```python
from build123d import *

# Parameters (mm, degrees)
EXTRUDE_1_DEPTH     = 3
SKETCH_2_R          = 1.6
CUT_EXTRUDE_1_DEPTH = 26.184320519
SKETCH_4_W          = 14
SKETCH_4_H          = 8
EXTRUDE_2_DEPTH     = 14.55
SKETCH_5_W          = 8
SKETCH_5_H          = 14.55
CUT_EXTRUDE_2_DEPTH = 32.452384647
SKETCH_6_R          = 1.05
CUT_EXTRUDE_3_DEPTH = 37.404017635
FILLET_1_R          = 3
RIB_1_REACH         = 32.549
SKETCH_7_WALL_W     = 71.642367062
SKETCH_7_WALL_H     = 3
RIB_2_REACH         = 32.549
SKETCH_8_WALL_W     = 71.642367062
SKETCH_8_WALL_H     = 3


with BuildPart() as part:
    # 草图1 → 凸台-拉伸1 (new body)
    with BuildSketch(Plane.XY):
        with BuildLine():
            Line((-21.779069767, 2.986991809), (-0.465116279, 4.978319681))
            ThreePointArc((-0.465116279, 4.978319681), (0, 5), (0.465116279, 4.978319681))
            Line((0.465116279, 4.978319681), (21.779069767, 2.986991809))
            ThreePointArc((21.779069767, 2.986991809), (24.5, 0), (21.779069767, -2.986991809))
            Line((21.779069767, -2.986991809), (0.465116279, -4.978319681))
            ThreePointArc((0.465116279, -4.978319681), (0, -5), (-0.465116279, -4.978319681))
            Line((-0.465116279, -4.978319681), (-21.779069767, -2.986991809))
            ThreePointArc((-21.779069767, -2.986991809), (-24.5, 0), (-21.779069767, 2.986991809))
        make_face()
    extrude(amount=EXTRUDE_1_DEPTH)

    # 草图2 → 切除-拉伸1 (cut, through all)
    with BuildSketch(Plane.XY.offset(3)):
        with Locations((-20, 0)):
            Circle(SKETCH_2_R)
        with Locations((20, 0)):
            Circle(SKETCH_2_R)
    extrude(amount=-CUT_EXTRUDE_1_DEPTH, mode=Mode.SUBTRACT)

    # 草图4 → 凸台-拉伸2 (add)
    with BuildSketch(Plane.XY.offset(3)):
        Rectangle(SKETCH_4_W, SKETCH_4_H)
    extrude(amount=EXTRUDE_2_DEPTH)

    # 草图5 → 切除-拉伸2 (cut, through all)
    with BuildSketch(Plane(origin=(0, 4, 0), x_dir=(1, 0, 0), z_dir=(0, 1, 0))):
        with Locations((0, -10.275)):
            Rectangle(SKETCH_5_W, SKETCH_5_H)
    extrude(amount=-CUT_EXTRUDE_2_DEPTH, mode=Mode.SUBTRACT)

    # 草图6 → 切除-拉伸3 (cut, through all)
    with BuildSketch(Plane(origin=(7, 0, 0), x_dir=(0, 0, -1), z_dir=(1, 0, 0))):
        with Locations((-15.55, 0)):
            Circle(SKETCH_6_R)
    extrude(amount=-CUT_EXTRUDE_3_DEPTH, mode=Mode.SUBTRACT)

    # 圆角1
    fillet_1_edges = [part.edges().sort_by_distance(p)[0] for p in [
        (-5.5, -4, 17.55),
        (5.5, 4, 17.55),
        (5.5, -4, 17.55),
        (-5.5, 4, 17.55),
    ]]
    fillet(fillet_1_edges, radius=FILLET_1_R)

    # 草图7 wall → 筋1 (add, up to next)
    with BuildSketch(Plane(origin=(8.5, 0, 7), x_dir=(-0.351123441588, 0, 0.936329177569), z_dir=(0.936329177569, 0, 0.351123441588)), mode=Mode.PRIVATE) as rib_1_sk1:
        Rectangle(SKETCH_7_WALL_W, SKETCH_7_WALL_H)
    rib_1_tool1 = extrude(rib_1_sk1.sketch, amount=-RIB_1_REACH, mode=Mode.PRIVATE) - part.part
    add(rib_1_tool1.solids().sort_by_distance((8.5, 0, 7))[0])

    # 草图8 wall → 筋2 (add, up to next)
    with BuildSketch(Plane(origin=(-8.5, 0, 7), x_dir=(0.351123441588, 0, 0.936329177569), z_dir=(0.936329177569, 0, -0.351123441588)), mode=Mode.PRIVATE) as rib_2_sk1:
        Rectangle(SKETCH_8_WALL_W, SKETCH_8_WALL_H)
    rib_2_tool1 = extrude(rib_2_sk1.sketch, amount=RIB_2_REACH, mode=Mode.PRIVATE) - part.part
    add(rib_2_tool1.solids().sort_by_distance((-8.5, 0, 7))[0])


solid = part.part
```
The model under review builds one solid part; all positions refer to its coordinate system, in mm. A direction names the side the tool comes from. Round coordinates to 2 decimals unless told otherwise and drop trailing zeros. Write each loop counter-clockwise with the first axis right and the second up, starting at its lowest first coordinate (ties: lowest second). Pieces come first, ordered by that corner, then holes. Notation, with made-up numbers: (-25, 43) - (-21, 43) arc R26 cw to (-21, 66) - close; hole circle Ø8 at (-7, 51). An arc over 180 degrees is marked (long way). Answer as CSV lines item,"result". Start each with the question number.
(1) We need section A-A on y = 0. Give the number of separate pieces and of enclosed holes in the cut face, plus the area to 4 significant figures.
(2) Draft analysis for pull direction Y (two halves, no side actions). For faces 1 (the cylindrical face through (-5.5, 0, 16.6)), 2 (the flat face through (8, 1.5, 6)), 3 (the cylindrical face through (-21.18, 1.08, 1.52)), 4 (the flat face through (-10.973, -3.997, 1.479)), state which applies: pulls with the +Y half, pulls with the -Y half, needs draft (parallel to the pull), parting line crosses it, or undercut.
(3) We need section D-D on x = 6.5. State the section outline as (y, z) points, plus the area to 3 significant figures.
(4) For faces 5 (the flat face through (4, 0, 10)), 6 (the flat face through (5, -4, 9)), 7 (the flat face through (7, 0, 12)), 8 (the flat face through (-8, -1.5, 6)), list the 3-axis set-ups (+Z, -Z, +X, -X, +Y, -Y) from which the entire face can be reached by the end or side of a thin tool; tool diameter is ignored.
(5) To check wall thickness, follow line 1 (X direction, y = 1.25, z = 1); line 2 (X direction, y = 0.75, z = 1); line 3 (X direction, y = -3.75, z = 13). State the ranges of each line that lie inside material, in increasing order.
(6) We need section C-C on z = 15.55. State the section outline as (x, y) points, plus the area to 3 significant figures.
(7) We need section B-B on x = 20. State the section outline as (y, z) points.
(8) For pin 1 Ø3 at (x, y) = (-3, -0.5) entering from +Z; pin 2 Ø2 at (x, z) = (-3.5, 3) entering from +Y; pin 3 Ø2.5 at (x, z) = (-5, 6) entering from +Y; pin 4 Ø8 at (x, z) = (10, 3) entering from +Y, all flat-tipped, find the tip position at first contact; note any pin that passes through.
Worked answers:
1,separate pieces,"5"
1,enclosed holes,"0"
1,area,"226.5 mm²"
2,face 1,"undercut"
2,face 2,"pulls with the +Y half"
2,face 3,"undercut"
2,face 4,"pulls with the -Y half"
3,outline,"(-4.41, 0) - (4.41, 0) - (4.41, 3) - (4, 3) - (4, 14.55) arc R3 ccw to (1, 17.55) - (-1, 17.55) arc R3 ccw to (-4, 14.55) - (-4, 3) - (-4.41, 3) - close; hole circle Ø2.1 at (0, 15.55)"
3,area,"136 mm²"
4,face 5,"+Z, +Y, -Y"
4,face 6,"+Z, +X, -X, -Y"
4,face 7,"+Z, +X"
4,face 8,"+Z, -X, -Y"
5,line 1,"-24.23 to -21, -19 to 19, 21 to 24.23"
5,line 2,"-24.4 to -21.41, -18.59 to 18.59, 21.41 to 24.4"
5,line 3,"-7 to -4, 4 to 7"
6,outline,"(-7, -3.83) - (-4, -3.83) - (-4, -1.05) - (-7, -1.05) - close; (-7, 1.05) - (-4, 1.05) - (-4, 3.83) - (-7, 3.83) - close; (4, -3.83) - (7, -3.83) - (7, -1.05) - (4, -1.05) - close; (4, 1.05) - (7, 1.05) - (7, 3.83) - (4, 3.83) - close"
6,area,"33.3 mm²"
7,outline,"(-3.15, 0) - (-1.6, 0) - (-1.6, 3) - (-3.15, 3) - close; (1.6, 0) - (3.15, 0) - (3.15, 3) - (1.6, 3) - close"
8,pin 1,"z = 17.55"
8,pin 2,"y = 4.79"
8,pin 3,"y = 4"
8,pin 4,"y = 4.46"
